The figure shows three views and two pictorial views of one solid part (mm, origin at its lowest corner). Answer the questions. Round coordinates to 2 decimals unless told otherwise and drop trailing zeros. Order: outer loops, then holes, each group sorted by start corner. A loop starts at its lowest first (then second) coordinate and runs counter-clockwise, first axis right, second up. Notation, with made-up numbers: (50.5, 89.5) - (89.5, 89.5) arc R25 ccw to (89.5, 122.5) - close; hole circle Ø1 at (59, 29.25). An arc over 180 degrees is marked (long way). Use CSV: the item, a comma, the result in double quotes.
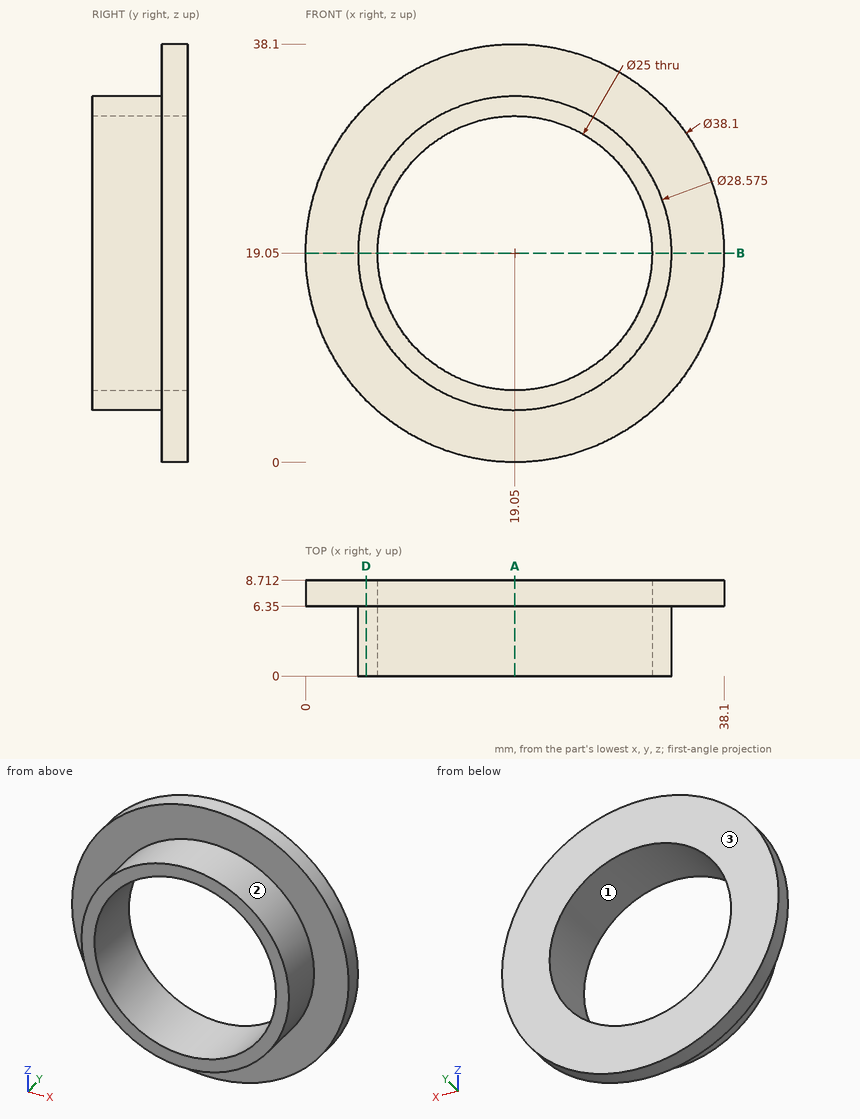
(1) The mould has two halves that part along X. Classify the marked faces 1, 2 and 3: released by +X, released by -X, zero draft, split by the parting line, or undercut.
Findings below:
face 1,"undercut"
face 2,"split by the parting line"
face 3,"zero draft"
(2) Find section A-A (x = 19.05). Determine the outline of the cut face in (y, z).
Findings below:
outline,"(0, 4.76) - (6.35, 4.76) - (6.35, 0) - (8.71, 0) - (8.71, 6.55) - (0, 6.55) - close; (0, 31.55) - (8.71, 31.55) - (8.71, 38.1) - (6.35, 38.1) - (6.35, 33.34) - (0, 33.34) - close"
(3) Find section B-B (z = 19.05). Determine the outline of the cut face in (x, y).
Findings below:
outline,"(0, 6.35) - (4.76, 6.35) - (4.76, 0) - (6.55, 0) - (6.55, 8.71) - (0, 8.71) - close; (31.55, 0) - (33.34, 0) - (33.34, 6.35) - (38.1, 6.35) - (38.1, 8.71) - (31.55, 8.71) - close"
(4) Find section D-D (x = 5.5). Determine the outline of the cut face in (y, z).
Findings below:
outline,"(0, 14.52) - (6.35, 14.52) - (6.35, 5.66) - (8.71, 5.66) - (8.71, 32.44) - (6.35, 32.44) - (6.35, 23.58) - (0, 23.58) - close"
(5) Find the intervals of material crossed by L1, parallel to Z at x = 19.05, y = 6.5; L2, parallel to Z at x = 19.05, y = 2.5, in increasing order. Write a range as from..to.
Findings below:
L1,"z = 0..6.55, 31.55..38.1"
L2,"z = 4.76..6.55, 31.55..33.34"
(6) Each of these flat-tipped pins is pushed along its axis until it touches: pin 1 (5 mm diameter, centred on x = 21, y = 6.5, fed in from -Z); pin 2 (4 mm diameter, centred on x = 26, y = 6.5, fed in from +Z); pin 3 (2 mm diameter, centred on y = 3.5, z = 27.5, fed in from +X); pin 4 (10 mm diameter, centred on x = 17, z = 11.5, fed in from +Y). Where does it stop, or does it pass through?
Findings below:
pin 1,"stops at z = 0"
pin 2,"stops at z = 37.45"
pin 3,"stops at x = 31.24"
pin 4,"stops at y = 8.71"
